from build123d import *

# Parameters (mm, degrees)
F0_R     = 9.5
F0_R_2   = 4
F1_DEPTH = 6


with BuildPart() as f1:
    # F0 (on Front) → F1 (new body)
    with BuildSketch(Plane.XZ):
        with BuildLine():
            ThreePointArc((2.350153171, 12.7858038493), (1.1720328397, 12.8595060447), (0, 13))
            ThreePointArc((0, 13), (-11.2995091051, -6.4281485658), (11.1746035767, -6.6429086178))
            ThreePointArc((11.1746035767, -6.6429086178), (12.5353469536, -3.4445720709), (13, 0))
            ThreePointArc((13, 0), (9.9887935013, 8.320096417), (2.350153171, 12.7858038493))
        make_face()
        Circle(F0_R, mode=Mode.SUBTRACT)
        with BuildLine():
            ThreePointArc((2.350153171, 12.7858038493), (1.179947024, 12.9463402172), (0, 13))
            ThreePointArc((0, 13), (1.1720328397, 12.8595060447), (2.350153171, 12.7858038493))
        make_face()
        with BuildLine():
            ThreePointArc((13, 0), (12.5353469536, -3.4445720709), (11.1746035767, -6.6429086178))
            ThreePointArc((11.1746035767, -6.6429086178), (20.3927051131, 2.2823011589), (32.8593572911, 5.3179804839))
            ThreePointArc((32.8593572911, 5.3179804839), (22.0397803989, 11.649441895), (21.5996059124, 24.1776857522))
            ThreePointArc((21.5996059124, 24.1776857522), (13.63881463, 15.6701075209), (2.350153171, 12.7858038493))
            ThreePointArc((2.350153171, 12.7858038493), (9.9887935013, 8.320096417), (13, 0))
        make_face()
        with BuildLine():
            ThreePointArc((21.5996059124, 24.1776857522), (22.0397803989, 11.649441895), (32.8593572911, 5.3179804839))
            ThreePointArc((32.8593572911, 5.3179804839), (42.272310005, 9.0007955279), (46.2018025219, 18.3134693652))
            ThreePointArc((46.2018025219, 18.3134693652), (45.8389012751, 21.3636718342), (44.7704586601, 24.243578568))
            ThreePointArc((44.7704586601, 24.243578568), (33.1648335269, 31.3134167995), (21.5996059124, 24.1776857522))
        make_face()
        with BuildLine():
            ThreePointArc((46.2018025219, 18.3134693652), (42.272310005, 9.0007955279), (32.8593572911, 5.3179804839))
            ThreePointArc((32.8593572911, 5.3179804839), (44.5354086005, 1.9994233392), (53.1813680275, -6.5205755628))
            ThreePointArc((53.1813680275, -6.5205755628), (52.7786540902, 6.1760009355), (63.3931152108, 13.154428295))
            ThreePointArc((63.3931152108, 13.154428295), (52.487300782, 16.0212898755), (44.7704586601, 24.243578568))
            ThreePointArc((44.7704586601, 24.243578568), (45.8389012751, 21.3636718342), (46.2018025219, 18.3134693652))
        make_face()
        with BuildLine():
            ThreePointArc((21.5996059834, 42.9212888668), (23.8334826654, 33.549487301), (21.5996059124, 24.1776857522))
            ThreePointArc((21.5996059124, 24.1776857522), (33.1648335269, 31.3134167995), (44.7704586601, 24.243578568))
            ThreePointArc((44.7704586601, 24.243578568), (42.5243018444, 33.5494874141), (44.7704586914, 42.8553962526))
            ThreePointArc((44.7704586914, 42.8553962526), (40.2259887899, 37.846547159), (33.7803843902, 35.7983870449))
            ThreePointArc((33.7803843902, 35.7983870449), (33.7804919256, 35.7919466185), (33.7805277722, 35.7855053943))
            ThreePointArc((33.7805277722, 35.7855053943), (33.1953612977, 35.2068159906), (32.6232206536, 35.7983870449))
            ThreePointArc((32.6232206536, 35.7983870449), (26.1465368827, 37.8665664916), (21.5996059834, 42.9212888668))
        make_face()
        with BuildLine():
            ThreePointArc((63.3931152108, 13.154428295), (52.7786540902, 6.1760009355), (53.1813680275, -6.5205755628))
            ThreePointArc((53.1813680275, -6.5205755628), (67.7981541622, -12.3379567831), (77.3170911302, 0.1873056959))
            ThreePointArc((77.3170911302, 0.1873056959), (73.176783931, 9.7007616124), (63.3931152108, 13.154428295))
        make_face()
        with Locations((64.3170911302, 0.1873056959)):
            Circle(F0_R, mode=Mode.SUBTRACT)
        with BuildLine():
            ThreePointArc((46.2018025219, 48.7855053943), (30.1875492977, 61.4312271017), (21.5996059834, 42.9212888668))
            ThreePointArc((21.5996059834, 42.9212888668), (26.1465368827, 37.8665664916), (32.6232206536, 35.7983870449))
            ThreePointArc((32.6232206536, 35.7983870449), (33.2018025219, 36.3642306445), (33.7803843902, 35.7983870449))
            ThreePointArc((33.7803843902, 35.7983870449), (40.2259887899, 37.846547159), (44.7704586914, 42.8553962526))
            ThreePointArc((44.7704586914, 42.8553962526), (45.8389012832, 45.7353029587), (46.2018025219, 48.7855053943))
        make_face()
        with Locations((33.2018025219, 48.7855053943)):
            Circle(F0_R, mode=Mode.SUBTRACT)
        with Locations((33.2018025219, 48.7855053943)):
            Circle(F0_R)
        with Locations((33.2018025219, 48.7855053943)):
            Circle(F0_R_2, mode=Mode.SUBTRACT)
        Circle(F0_R)
        Circle(F0_R_2, mode=Mode.SUBTRACT)
        with Locations((64.3170911302, 0.1873056959)):
            Circle(F0_R)
        with Locations((64.3170911302, 0.1873056959)):
            Circle(F0_R_2, mode=Mode.SUBTRACT)
    extrude(amount=F1_DEPTH)


solid = f1.part
Model file for the job. Use its own axes, mm. Give positions to 0.01 mm unless a question says otherwise; leave off trailing zeros. Loops run counter-clockwise (first coordinate to the right, second up) from the corner with the lowest first, then second, coordinate; pieces in that order, holes last.
1) Saw through at B-B (x = 5.5). Write the cut outline in (y, z), plus the area to 3 significant figures.
2) Wall check: line 1 (X direction, y = -3.3, z = -2.5); line 2 (Z direction, x = 62, y = -5.65); line 3 (Z direction, x = 0, y = -4.35). Give the ranges that are in metal, low to high.
3) Saw through at C-C (z = 16). Write the cut outline in (x, y), plus the area to 3 significant figures.
4) Saw through at A-A (y = -2.2). Write the cut outline in (x, z).
5) Flat gauge pins, fed straight in: pin 1 Ø9 at (x, z) = (64.32, 0.19) entering from +Y; pin 2 Ø5 at (x, z) = (33.2, 48.79) entering from +Y; pin 3 Ø2 at (y, z) = (-0.5, -2.5) entering from +X. Where does each tip first touch, or does it go through?
6) Pull direction Z, two halves, no side cores. Call faces 1 (the cylindrical face through (30.254, -2.958, 51.489)), 2 (the cylindrical face through (75.673, -2.958, -6.141)), 3 (the flat face through (32, 0, 17)): +Z half, -Z half, draft (parallel to the pull), parting line (faces both ways), or undercut.
Answer block:
1. outline: (-6, -11.78) - (0, -11.78) - (0, 12.92) - (-6, 12.92) - close
1. area: 148 mm2
2. line 1: x = -12.76 to -3.12, 3.12 to 14.27, 50.16 to 61.35, 67.28 to 77.04
2. line 2: z = -12.6 to -3.07, 3.45 to 13.17
2. line 3: z = -13 to -4, 4 to 13
3. outline: (14.18, -6) - (52.52, -6) - (52.52, 0) - (14.18, 0) - close
3. area: 230 mm2
4. outline: (2.35, 12.79) arc R13 ccw (long way) to (11.17, -6.64) arc R24.48 cw to (53.18, -6.52) arc R13 ccw (long way) to (63.39, 13.15) arc R20.4 cw to (44.77, 42.86) arc R13 ccw (long way) to (21.6, 42.92) arc R20.78 cw to start; hole circle Ø8 at (0, 0); hole circle Ø8 at (33.2, 48.79); hole circle Ø1.16 at (33.2, 35.79); hole circle Ø8 at (64.32, 0.19)
5. pin 1: stops at y = 0
5. pin 2: passes through
5. pin 3: stops at x = 77.21
6. face 1: undercut
6. face 2: parting line
6. face 3: draft
